from build123d import *

# Parameters (mm, degrees)
SKETCH1_W           = 37.2
SKETCH1_H           = 32.1
BOSS_EXTRUDE1_DEPTH = 34.1
SKETCH1_4_W         = 43.2
SKETCH1_4_H         = 38.1
SKETCH1_4_W_2       = 37.2
SKETCH1_4_H_2       = 32.1
BOSS_EXTRUDE2_DEPTH = 12.7
BOSS_EXTRUDE3_START = 1
SKETCH2_R           = 3.5
BOSS_EXTRUDE3_DEPTH = 2.5


with BuildPart() as part:
    # Sketch1 → Boss-Extrude1 (new body)
    with BuildSketch(Plane(origin=(0, 0, 0), x_dir=(1, 0, 0), z_dir=(0, 1, 0))):
        Rectangle(SKETCH1_W, SKETCH1_H)
    extrude(amount=BOSS_EXTRUDE1_DEPTH)

    # Sketch1_4 → Boss-Extrude2 (add)
    with BuildSketch(Plane(origin=(0, 0, 0), x_dir=(1, 0, 0), z_dir=(0, 1, 0))):
        Rectangle(SKETCH1_4_W, SKETCH1_4_H)
        Rectangle(SKETCH1_4_W_2, SKETCH1_4_H_2, mode=Mode.SUBTRACT)
    extrude(amount=BOSS_EXTRUDE2_DEPTH)

    # Sketch2 → Boss-Extrude3 (add)
    with BuildSketch(Plane(origin=(0, 0, 0), x_dir=(1, 0, 0), z_dir=(0, 1, 0)).offset(BOSS_EXTRUDE3_START)):
        Polygon((-21.6, 1.45), (-40.5, 1.45), (-42.5, -0.55), (-42.5, -14.55), (-40.5, -16.55), (-21.6, -16.55), align=None)
        with Locations((-30, -7.55)):
            Circle(SKETCH2_R, mode=Mode.SUBTRACT)
        Polygon((21.6, -16.55), (40.5, -16.55), (42.5, -14.55), (42.5, -0.55), (40.5, 1.45), (21.6, 1.45), align=None)
        with Locations((30, -7.55)):
            Circle(SKETCH2_R, mode=Mode.SUBTRACT)
    extrude(amount=BOSS_EXTRUDE3_DEPTH)


solid = part.part
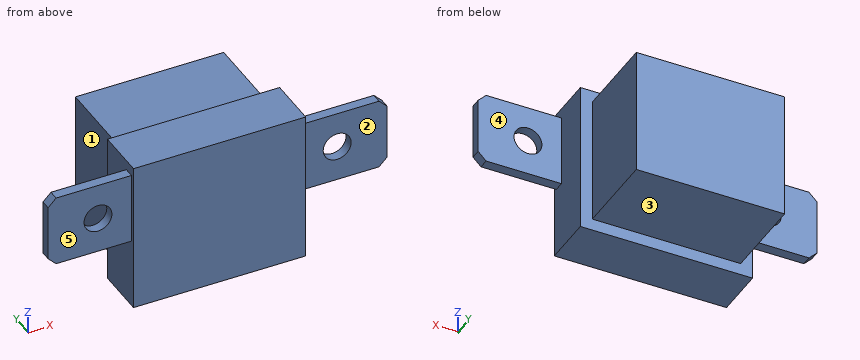
Work out the finished part from the listing and answer in its coordinate system (mm). Face numbers are marked on the shaded views. A direction names the side the tool comes from. Give positions to 0.01 mm unless a question says otherwise; leave off trailing zeros. Order: outer loops, then holes, each group sorted by start corner. A loop starts at its lowest first (then second) coordinate and runs counter-clockwise, first axis right, second up. Notation, with made-up numbers: (87.5, 47.5) -> (100.5, 47.5) arc R32 ccw to (100.5, 81.5) -> close; hole circle Ø2 at (17, 34.25). An arc over 180 degrees is marked (long way). Answer as a JSON object with one key per item and string values. Group by question number.
1. A tool of negligible diameter and unlimited length cuts with its end or side. For the marked faces 1, 2, 3, 4 and 5, from which of +Z, -Z, +X, -X, +Y, -Y can it reach the whole face along a straight path? Write none if from no direction.
2. Section D-D on x = -11 is taken. Determine the outline of the cut face in (y, z), plus the area to 3 significant figures.
3. Section C-C on z = -8 is taken. Determine the outline of the cut face in (x, y).
4. Section A-A on x = -30 is taken. Determine the outline of the cut face in (y, z).
5. Consider line 1 along X through (y, z) = (2.35, 7.55); line 2 along Z through (x, y) = (30, 2); line 3 along Y through (x, z) = (32, 3.5). Determine where each line is inside the solid, lowest interval first. Write a range as [from, to].
6. Flat-ended cylindrical pins translate along their axes: pin 1 Ø6.5 at (x, y) = (-2.5, 26.5) entering from +Z; pin 2 Ø14.5 at (x, z) = (-31, 10) entering from +Y; pin 3 Ø0.8 at (x, y) = (33, 2.5) entering from +Z; pin 4 Ø4 at (x, z) = (30, 7.55) entering from -Y. Find the tip coordinate at first contact, or state that the pin passes through.
7. Section B-B on z = 7.55 is taken. Determine the outline of the cut face in (x, y).
Result sheet:
{
 "1": {"face 1": "+Z, -Z, -X, +Y", "face 2": "+Z, -Z, +X, -Y", "face 3": "-Z, +X, -X, +Y", "face 4": "+Z, -Z, +X, +Y", "face 5": "+Z, -Z, -X, -Y"},
 "2": {"outline": "(0, -19.05) -> (12.7, -19.05) -> (12.7, -16.05) -> (34.1, -16.05) -> (34.1, 16.05) -> (12.7, 16.05) -> (12.7, 19.05) -> (0, 19.05) -> close", "area": "1,170 mm^2"},
 "3": {"outline": "(-21.6, 0) -> (21.6, 0) -> (21.6, 12.7) -> (18.6, 12.7) -> (18.6, 34.1) -> (-18.6, 34.1) -> (-18.6, 12.7) -> (-21.6, 12.7) -> close"},
 "4": {"outline": "(1, -1.45) -> (3.5, -1.45) -> (3.5, 4.05) -> (1, 4.05) -> close; (1, 11.05) -> (3.5, 11.05) -> (3.5, 16.55) -> (1, 16.55) -> close"},
 "5": {"line 1": "x = [-42.5, -33.5], [-26.5, 26.5], [33.5, 42.5]", "line 2": "z = [-1.45, 4.05], [11.05, 16.55]", "line 3": "y = [1, 3.5]"},
 "6": {"pin 1": "stops at z = 16.05", "pin 2": "stops at y = 3.5", "pin 3": "stops at z = 16.55", "pin 4": "passes through"},
 "7": {"outline": "(-42.5, 1) -> (-33.5, 1) -> (-33.5, 3.5) -> (-42.5, 3.5) -> close; (-26.5, 1) -> (-21.6, 1) -> (-21.6, 0) -> (21.6, 0) -> (21.6, 1) -> (26.5, 1) -> (26.5, 3.5) -> (21.6, 3.5) -> (21.6, 12.7) -> (18.6, 12.7) -> (18.6, 34.1) -> (-18.6, 34.1) -> (-18.6, 12.7) -> (-21.6, 12.7) -> (-21.6, 3.5) -> (-26.5, 3.5) -> close; (33.5, 1) -> (42.5, 1) -> (42.5, 3.5) -> (33.5, 3.5) -> close"}
}
